from build123d import *

# Parameters (mm, degrees)
F0_W     = 240
F0_H     = 59.62
F1_DEPTH = 16
F3_DEPTH = 240
F4_SIZE  = 15.99999


# Not quite as in the source:
# - a fillet or chamfer is up to 0.001 mm smaller than in the source, because OpenCascade refuses the exact size


with BuildPart() as f1:
    # F0 (on Front) → F1 (new body)
    with BuildSketch(Plane.XZ):
        with Locations((120, 29.81)):
            Rectangle(F0_W, F0_H)
    extrude(amount=F1_DEPTH)

    # F2 (on Right) → F3 (join)
    with BuildSketch(Plane.YZ):
        Polygon((0, 63.9071870789), (-16, 59.62), (0, 59.62), align=None)
    extrude(amount=F3_DEPTH)

    # F4 (size 16 in the source; OpenCascade refuses exactly that, so slightly less here)
    f4_edges = [f1.edges().sort_by_distance(p)[0] for p in [
        (0, 0, 31.953594),
        (120, 0, 0),
        (240, 0, 31.953594),
    ]]
    chamfer(f4_edges, length=F4_SIZE)


solid = f1.part
Could you check a few things on this model? Use its own coordinates, in mm. Coordinates: 2 decimals unless noted, no trailing zeros. Write each loop counter-clockwise with the first axis right and the second up, starting at its lowest first coordinate (ties: lowest second). Pieces come first, ordered by that corner, then holes. Notation, with made-up numbers: (37, 11) - (62, 11) arc R21 ccw to (62, 16) - close; hole circle Ø5 at (-3.5, 25). An arc over 180 degrees is marked (long way). Write item = value, one per line.
1) Suppose I cut it at C-C on y = -7.5. Please give me the cut outline in (x, z), plus the area to 3 significant figures.
Result set:
outline = (8.5, 8.5) - (231.5, 8.5) - (231.5, 61.9) - (8.5, 61.9) - close
area = 11,900 mm2
2) Will these pins go through, and if not, where does the flat tip stop? pin 1 Ø1.5 at (x, y) = (25.5, -7) entering from -Z; pin 2 Ø2 at (y, z) = (-7, 7.5) entering from +X; pin 3 Ø5 at (x, y) = (85.5, -6) entering from +Z; pin 4 Ø1 at (y, z) = (-11.5, 8.5) entering from +X.
Result set:
pin_1 = 8.25
pin_2 = through
pin_3 = 62.97
pin_4 = 236
3) Please list where these lines run through material, in increasing order: line 1 (Z direction, x = 186.5, y = -8.5); line 2 (X direction, y = -3, z = 19); line 3 (Z direction, x = 48, y = -4). Write a range as [from, to].
Result set:
line_1 = [7.5, 61.63]
line_2 = [13, 227]
line_3 = [12, 62.84]
